For this review, take the finished solid that the model builds, in its own axes (mm). A direction names the side the tool comes from. Round coordinates to 2 decimals unless told otherwise and drop trailing zeros. Order: outer loops, then holes, each group sorted by start corner. A loop starts at its lowest first (then second) coordinate and runs counter-clockwise, first axis right, second up. Notation, with made-up numbers: M 81,51 L 91,51 A11 cw 91,69 Z; hole C 75,19.25 d5. An arc over 180 degrees is marked long. Use a Markdown table: item, result.
from build123d import *

# Parameters (mm, degrees)
BOSS_EXTRUDE1_DEPTH   = 4.1275
CUT_EXTRUDE1_DEPTH    = 1.5875
F_4_40_TAPPED_HOLE1_D = 2.2606
BOSS_EXTRUDE2_DEPTH   = 1.5875
FILLET1_R             = 1.5875
FILLET2_R             = 0.8128
FILLET3_R             = 0.8128
FILLET4_R             = 0.8128


with BuildPart() as part:
    # Sketch1 → Boss-Extrude1 (new body)
    with BuildSketch(Plane.XY):
        with BuildLine():
            Line((-16.5735, 4.0005), (16.5735, 4.0005))
            ThreePointArc((16.5735, 4.0005), (20.574, 0), (16.5735, -4.0005))
            Line((16.5735, -4.0005), (-16.5735, -4.0005))
            ThreePointArc((-16.5735, -4.0005), (-20.574, 0), (-16.5735, 4.0005))
        make_face()
    extrude(amount=BOSS_EXTRUDE1_DEPTH)

    # Sketch2 → Cut-Extrude1 (cut)
    with BuildSketch(Plane.XY.offset(4.1275)):
        with BuildLine():
            Line((-10.9855, 1.5875), (10.9855, 1.5875))
            ThreePointArc((10.9855, 1.5875), (12.573, 0), (10.9855, -1.5875))
            Line((10.9855, -1.5875), (-10.9855, -1.5875))
            ThreePointArc((-10.9855, -1.5875), (-12.573, 0), (-10.9855, 1.5875))
        make_face()
    extrude(amount=-CUT_EXTRUDE1_DEPTH, mode=Mode.SUBTRACT)

    # #4-40 Tapped Hole1 (through all)
    with Locations(Plane.XY.offset(4.1275)):
        with Locations((-16.5735, 0), (16.5735, 0)):
            Hole(F_4_40_TAPPED_HOLE1_D / 2)

    # Sketch5 → Boss-Extrude2 (add, symmetric)
    with BuildSketch(Plane(origin=(0, 0, 0), x_dir=(1, 0, 0), z_dir=(0, 1, 0))):
        Polygon((-12.573, 0), (-12.573, 6.985), (-10.9855, 6.985), (-7.9375, 3.175), (7.9375, 3.175), (10.9855, 6.985), (12.573, 6.985), (12.573, 0), align=None)
    extrude(amount=BOSS_EXTRUDE2_DEPTH, both=True)

    # Fillet1
    fillet1_edges = [part.edges().sort_by_distance(p)[0] for p in [
        (10.9855, 0, -6.985),
        (7.9375, 0, -3.175),
        (-7.9375, 0, -3.175),
        (-10.9855, 0, -6.985),
    ]]
    fillet(fillet1_edges, radius=FILLET1_R)

    # Fillet2
    fillet2_edges = [part.edges().sort_by_distance(p)[0] for p in [
        (12.573, -1.5875, -3.4925),
        (-12.573, -1.5875, -3.4925),
        (12.573, 1.5875, -3.4925),
        (-12.573, 1.5875, -3.4925),
    ]]
    fillet(fillet2_edges, radius=FILLET2_R)

    # Fillet3
    fillet3_edges = [part.edges().sort_by_distance(p)[0] for p in [
        (12.573, 0, 0),
        (11.754345973, -1.5875, -6.985),
        (11.754345973, 1.5875, -6.985),
        (12.334936392, 1.349436392, -6.985),
        (12.334936392, -1.349436392, -6.985),
        (0, -1.5875, 0),
        (0, 1.5875, 0),
        (-12.573, 0, 0),
        (-12.573, 0, -6.985),
        (-12.334936392, 1.349436392, -6.985),
        (-12.334936392, -1.349436392, -6.985),
        (12.334936392, -1.349436392, 0),
        (12.334936392, 1.349436392, 0),
        (-12.334936392, -1.349436392, 0),
        (-12.334936392, 1.349436392, 0),
        (-20.574, 0, 4.1275),
        (0, -4.0005, 4.1275),
        (12.573, 0, 4.1275),
        (0, 1.5875, 4.1275),
        (-12.573, 0, 4.1275),
        (0, -1.5875, 4.1275),
        (20.574, 0, 4.1275),
        (-11.754345973, -1.5875, -6.985),
        (-11.754345973, 1.5875, -6.985),
        (-9.4615, -1.5875, -5.08),
        (0, -1.5875, -3.175),
        (9.4615, -1.5875, -5.08),
        (11.060804836, -1.5875, -6.828318888),
        (-11.060804836, -1.5875, -6.828318888),
        (-9.4615, 1.5875, -5.08),
        (9.4615, 1.5875, -5.08),
        (0, 1.5875, -3.175),
        (11.060804836, 1.5875, -6.828318888),
        (-11.060804836, 1.5875, -6.828318888),
        (7.862195164, -1.5875, -3.331681112),
        (7.862195164, 1.5875, -3.331681112),
        (-7.862195164, -1.5875, -3.331681112),
        (-7.862195164, 1.5875, -3.331681112),
        (0, 4.0005, 4.1275),
        (12.573, 0, -6.985),
    ]]
    fillet(fillet3_edges, radius=FILLET3_R)

    # Fillet4
    # the kernel refuses this fillet: 0.8128 mm, written as the material it adds along each edge
    with BuildSketch(Plane(origin=(10.9855, -1.5875, 2.54), x_dir=(0, -0.00028128862329323027, 0.9999999604383545), z_dir=(-1, 0, 0)), Plane(origin=(-10.9855, 1.5875, 2.54), x_dir=(0, 0.00028128862329323027, 0.9999999604383545), z_dir=(1, 0, 0))) as fillet4_piece_1:
        with BuildLine():
            CenterArc((0.812571462, 0.812582054), FILLET4_R, 180.016116651, 88.657007194)
            Line((-0.000228506, 0.812353422), (-0.081508503, 0.812330559))
            Line((-0.081508503, 0.812330559), (-0.081279997, -2.2863e-05))
            Line((-0.081279997, -2.2863e-05), (2.2863e-05, -0.081279997))
            ThreePointArc((2.2863e-05, -0.081279997), (0.774722832, -0.081062082), (0.791867888, -0.081258205))
            Line((0.791867888, -0.081258205), (0.793750031, 0))
        make_face()
    extrude(amount=21.971)
    with BuildSketch(Plane(origin=(-10.9855, 0, 2.54), x_dir=(0, -1, 0), z_dir=(1, 0, 0))) as fillet4_piece_2:
        with BuildLine():
            CenterArc((0.775146546, -0.8128), FILLET4_R, 1.342992806, 88.657007194)
            Line((0.775146546, 0), (0.775146546, 0.08128))
            Line((0.775146546, 0.08128), (1.5875, 0.08128))
            Line((1.5875, 0.08128), (1.66878, 0))
            ThreePointArc((1.66878, 0), (1.66878, -0.7747), (1.668980946, -0.791845))
            Line((1.668980946, -0.791845), (1.587723273, -0.79375))
        make_face()
    revolve(axis=Axis((-10.9855, 0, 2.54), (0, 0, -1)), revolution_arc=180)
    with BuildSketch(Plane(origin=(10.9855, 0, 2.54), x_dir=(0, 1, 0), z_dir=(-1, 0, 0))) as fillet4_piece_3:
        with BuildLine():
            CenterArc((0.775146546, -0.8128), FILLET4_R, 1.342992806, 88.657007194)
            Line((0.775146546, 0), (0.775146546, 0.08128))
            Line((0.775146546, 0.08128), (1.5875, 0.08128))
            Line((1.5875, 0.08128), (1.66878, 0))
            ThreePointArc((1.66878, 0), (1.66878, -0.7747), (1.668980946, -0.791845))
            Line((1.668980946, -0.791845), (1.587723273, -0.79375))
        make_face()
    revolve(axis=Axis((10.9855, 0, 2.54), (0, 0, -1)), revolution_arc=180)


solid = part.part
Q1. Machinability: for faces 1 (the flat face through (12.573, 0, -4)), 2 (the cylindrical face through (-0.1, 1.343, -2.943)), 3 (the flat face through (0, 0, -3.175)), 4 (the cylindrical face through (-9.63, -1.34, -4.92)), 5 (the flat face through (0, -3, 0)), which of the approach directions +Z, -Z, +X, -X, +Y, -Y give a long, thin tool a straight path to every point of the face, cutting with its end or side? Answer none if there is none.
Determined:
| item | result |
|---|---|
| face 1 | -Z, +X, +Y, -Y |
| face 2 | -Z, +Y |
| face 3 | -Z, +Y, -Y |
| face 4 | -Z, -Y |
| face 5 | -Z |
Q2. Add section B-B (z = -1.25). Write out the cut boundary in (x, y).
Determined:
| item | result |
|---|---|
| outline | M -12.57,-0.77 A0.81 ccw -11.76,-1.59 L 11.76,-1.59 A0.81 ccw 12.57,-0.77 L 12.57,0.77 A0.81 ccw 11.76,1.59 L -11.76,1.59 A0.81 ccw -12.57,0.77 Z |
Q3. Add section A-A (x = 0.5). Write out the cut boundary in (y, z) (1 decimal), then the cut area to 3 significant figures.
Determined:
| item | result |
|---|---|
| outline | M -4,0 L -2.4,0 A0.8 cw -1.6,-0.8 L -1.6,-2.4 A0.8 ccw -0.8,-3.2 L 0.8,-3.2 A0.8 ccw 1.6,-2.4 L 1.6,-0.8 A0.8 cw 2.4,0 L 4,0 L 4,3.3 A0.8 ccw 3.2,4.1 L 2.4,4.1 A0.8 ccw 1.6,3.3 A0.8 cw 0.8,2.5 L -0.8,2.5 A0.8 cw -1.6,3.3 A0.8 ccw -2.4,4.1 L -3.2,4.1 A0.8 ccw -4,3.3 Z |
| area | 37.8 mm^2 |
Q4. Wall thickness on line 1 along X through (y, z) = (1, 2.25); line 2 along Z through (x, y) = (13, 1.75); line 3 along X through (y, z) = (-3.25, 1.75): over which ranges is each line inside the solid? List them lowest first. Write a range as [from, to].
Determined:
| item | result |
|---|---|
| line 1 | x = [-20.45, -17.1], [-16.05, 16.05], [17.1, 20.45] |
| line 2 | z = [0, 4.13] |
| line 3 | x = [-18.91, 18.91] |
Q5. Clearance check with flat-ended pins moving along their axes: pin 1 (1.2 mm diameter, centred on x = 3, y = 0, fed in from -Z) (3 decimals); pin 2 (6 mm diameter, centred on x = -1, z = -4, fed in from -Y); pin 3 (1 mm diameter, centred on x = 5.5, y = -0.5, fed in from +Z); pin 4 (2 mm diameter, centred on x = -16.57, y = 0, fed in from -Z). State where each tip first meets the part, or that it passes through.
Determined:
| item | result |
|---|---|
| pin 1 | stops at z = -3.175 |
| pin 2 | stops at y = -1.59 |
| pin 3 | stops at z = 2.57 |
| pin 4 | passes through |
Q6. Add section C-C (y = 0). Give the number of separate pieces and of enclosed holes in the cut face, then the cut area to 3 significant figures.
Determined:
| item | result |
|---|---|
| separate pieces | 3 |
| enclosed holes | 0 |
| area | 215 mm^2 |
